CAD build for the part. Positions are in the model's coordinates, mm. A direction names the side the tool comes from. Coordinates: 2 decimals unless noted, no trailing zeros. Write each loop counter-clockwise with the first axis right and the second up, starting at its lowest first coordinate (ties: lowest second). Pieces come first, ordered by that corner, then holes. Notation, with made-up numbers: (-13, -24) -> (25, -24) arc R17 cw to (25, -15) -> close; hole circle Ø1 at (37, 23). An arc over 180 degrees is marked (long way). Answer as CSV lines item,"result". Start each with the question number.
```python
from build123d import *

# Parameters (mm, degrees)
BOSS_EXTRUDE1_DEPTH = 20.32


with BuildPart() as part:
    # Sketch1 → Boss-Extrude1 (new body)
    with BuildSketch(Plane(origin=(0, 0, 0), x_dir=(1, 0, 0), z_dir=(0, 1, 0))):
        with BuildLine():
            Line((-2.286, 11.4935), (-2.286, 8.919207378))
            ThreePointArc((-2.286, 8.919207378), (0, 9.2075), (2.286, 8.919207378))
            Line((2.286, 8.919207378), (2.286, 11.4935))
            Line((2.286, 11.4935), (-2.286, 11.4935))
        make_face()
        with BuildLine():
            Line((-2.286, 8.919207378), (-2.286, 6.9215))
            Line((-2.286, 6.9215), (2.286, 6.9215))
            Line((2.286, 6.9215), (2.286, 8.919207378))
            ThreePointArc((2.286, 8.919207378), (0, 9.2075), (-2.286, 8.919207378))
        make_face()
        with BuildLine():
            Line((2.286, 6.9215), (-2.286, 6.9215))
            Line((-2.286, 6.9215), (-2.286, 8.919207378))
            ThreePointArc((-2.286, 8.919207378), (-9.2075, 0), (-2.286, -8.919207378))
            Line((-2.286, -8.919207378), (-2.286, -6.9215))
            Line((-2.286, -6.9215), (2.286, -6.9215))
            Line((2.286, -6.9215), (2.286, -8.919207378))
            ThreePointArc((2.286, -8.919207378), (7.274146041, -5.644896423), (9.2075, 0))
            ThreePointArc((9.2075, 0), (7.274146041, 5.644896423), (2.286, 8.919207378))
            Line((2.286, 8.919207378), (2.286, 6.9215))
        make_face()
        with BuildLine():
            Line((-2.286, -6.9215), (-2.286, -8.919207378))
            ThreePointArc((-2.286, -8.919207378), (0, -9.2075), (2.286, -8.919207378))
            Line((2.286, -8.919207378), (2.286, -6.9215))
            Line((2.286, -6.9215), (-2.286, -6.9215))
        make_face()
        with BuildLine():
            ThreePointArc((2.286, -8.919207378), (0, -9.2075), (-2.286, -8.919207378))
            Line((-2.286, -8.919207378), (-2.286, -11.4935))
            Line((-2.286, -11.4935), (2.286, -11.4935))
            Line((2.286, -11.4935), (2.286, -8.919207378))
        make_face()
    extrude(amount=BOSS_EXTRUDE1_DEPTH)


solid = part.part
```
1. Cut at B-B (x = -5.75). Give the cut face in (y, z), then the cut area to 3 significant figures.
2. Cut at A-A (y = 18.5). Give the cut face in (x, z) (1 decimal).
3. Wall check: line 1 (X direction, y = 19, z = 9); line 2 (Z direction, x = 6.5, y = 17.25); line 3 (X direction, y = 11.25, z = -5). Give the ranges that are in metal, low to high.
4. Flat gauge pins, fed straight in: P1, Ø1.3, axis at y = 15, z = -10.5, coming from the +X side; P2, Ø3, axis at x = 3, y = 9.5, coming from the -Z side; P3, Ø2, axis at y = 9, z = -10.5, coming from the -X side. Where does each tip first touch, or does it go through?
5. Cut at C-C (z = 2.5). Give the cut face in (x, y), then the cut area to 3 significant figures.
6. Tool access for faces 4 (the face through (-2.286, 10, -10)), 5 (the face through (2.286, 10, 10)), 6 (the face through (0, 10, -11.494)), 7 (the face through (-2.286, 10, 10)): list every direction of +Z, -Z, +X, -X, +Y, -Y with a clear straight run to the whole face (end or side of a thin tool).
7. Mould opens along X. For faces 1 (the face through (-9.206, 10.018, -0.17)), 2 (the face through (0, 20.32, 0)), 3 (the face through (2.286, 10, -10)) say: pulls with the +X half, pulls with the -X half, needs draft (parallel to the pull), parting line crosses it, or undercut.
Geometry check:
1,outline,"(0, -7.19) -> (20.32, -7.19) -> (20.32, 7.19) -> (0, 7.19) -> close"
1,area,"292 mm²"
2,outline,"(-2.3, -11.5) -> (2.3, -11.5) -> (2.3, -8.9) arc R9.2 ccw to (2.3, 8.9) -> (2.3, 11.5) -> (-2.3, 11.5) -> (-2.3, 8.9) arc R9.2 ccw to (-2.3, -8.9) -> close"
3,line 1,"-2.29 to 2.29"
3,line 2,"-6.52 to 6.52"
3,line 3,"-7.73 to 7.73"
4,P1,"x = 2.29"
4,P2,"z = -11.49"
4,P3,"x = -2.29"
5,outline,"(-8.86, 0) -> (8.86, 0) -> (8.86, 20.32) -> (-8.86, 20.32) -> close"
5,area,"360 mm²"
6,face 4,"-Z, -X, +Y, -Y"
6,face 5,"+Z, +X, +Y, -Y"
6,face 6,"-Z, +X, -X, +Y, -Y"
6,face 7,"+Z, -X, +Y, -Y"
7,face 1,"pulls with the -X half"
7,face 2,"needs draft"
7,face 3,"pulls with the +X half"
